from build123d import *

# Parameters (mm, degrees)
SKETCH1_W           = 17
SKETCH1_H           = 18.5
SKETCH1_R           = 1.5
BOSS_EXTRUDE1_DEPTH = 2
SKETCH3_R           = 0.325
LPATTERN1_COUNT     = 4
LPATTERN1_PITCH     = 2.54


with BuildPart() as part:
    # Sketch1 → Boss-Extrude1 (new body)
    with BuildSketch(Plane(origin=(0, 0, 0), x_dir=(1, 0, 0), z_dir=(0, 1, 0))):
        with Locations((8.5, 9.25)):
            Rectangle(SKETCH1_W, SKETCH1_H)
        with Locations(Location((2.5, 15.25, 0), (0, 0, 270))):
            Circle(SKETCH1_R, mode=Mode.SUBTRACT)
        with Locations(Location((2.5, 3.25, 0), (0, 0, 270))):
            Circle(SKETCH1_R, mode=Mode.SUBTRACT)
    extrude(amount=BOSS_EXTRUDE1_DEPTH)

    # Sweep1: sweep along a path in Sketch2
    with BuildLine(Plane.ZY.offset(-7)) as sweep1_path:
        Line((-1, -1), (-1, 3.5))
        ThreePointArc((-1, 3.5), (-0.853553391, 3.853553391), (-0.5, 4))
        Line((-0.5, 4), (29, 4))
    # Sketch3 → Sweep1 (sweep)
    with BuildSketch(Plane(origin=(0, 2, 0), x_dir=(1, 0, 0), z_dir=(0, 1, 0))):
        with Locations((7, 1)):
            Circle(SKETCH3_R)
    sweep1 = sweep(path=sweep1_path.line)

    # LPattern1: Sweep1 ×4
    with Locations(*[(i * LPATTERN1_PITCH, 0, 0) for i in range(1, LPATTERN1_COUNT)]):
        add(sweep1)


solid = part.part
Design review of the part built by this model. Coordinates are the model's own, in mm. Coordinates: 2 decimals unless noted, no trailing zeros. Order: outer loops, then holes, each group sorted by start corner. A loop starts at its lowest first (then second) coordinate and runs counter-clockwise, first axis right, second up. Notation, with made-up numbers: M 9.5,11 L 61.5,11 A27 ccw 61.5,49 Z; hole C -14,-35 d10. An arc over 180 degrees is marked long. Use a Markdown table: item, result.
(1) For P1, Ø3.5, axis at x = 2.5, z = -15.25, coming from the +Y side; P2, Ø1.5, axis at x = 13, z = 23, coming from the +Y side; P3, Ø6, axis at x = 5, z = -4, coming from the -Y side, all flat-tipped, find the tip position at first contact; note any pin that passes through.
Worked answers:
| item | result |
|---|---|
| P1 | stops at y = 2 |
| P2 | stops at y = 4.28 |
| P3 | stops at y = 0 |
(2) Wall thickness on probe 1 along X at (y, z) = (0.55, -3.25); probe 2 along X at (y, z) = (3.95, 7.5); probe 3 along Y at (x, z) = (15, -11): over which ranges is each line inside the solid? List them lowest first.
Worked answers:
| item | result |
|---|---|
| probe 1 | x = 0 to 1, 4 to 17 |
| probe 2 | x = 6.68 to 7.32, 9.22 to 9.86, 11.76 to 12.4, 14.3 to 14.94 |
| probe 3 | y = 0 to 2 |
(3) Add section A-A (x = 3.5). Give the boundary of the cut face in (y, z), then the cut area to 3 significant figures.
Worked answers:
| item | result |
|---|---|
| outline | M 0,-18.5 L 2,-18.5 L 2,-16.37 L 0,-16.37 Z; M 0,-14.13 L 2,-14.13 L 2,-4.37 L 0,-4.37 Z; M 0,-2.13 L 2,-2.13 L 2,0 L 0,0 Z |
| area | 28.1 mm2 |
(4) Add section B-B (z = -15.25). Give the boundary of the cut face in (x, y), then the cut area to 3 significant figures.
Worked answers:
| item | result |
|---|---|
| outline | M 0,0 L 1,0 L 1,2 L 0,2 Z; M 4,0 L 17,0 L 17,2 L 4,2 Z |
| area | 28.0 mm2 |
(5) Add section D-D (x = 7.75). Give the boundary of the cut face in (y, z), then the cut area to 3 significant figures.
Worked answers:
| item | result |
|---|---|
| outline | M 0,-18.5 L 2,-18.5 L 2,0 L 0,0 Z |
| area | 37.0 mm2 |
(6) Add section C-C (z = 25.5). Give the boundary of the cut face in (x, y) (3 decimals), then the cut area to 3 significant figures.
Worked answers:
| item | result |
|---|---|
| outline | C 7,4 d0.65; C 9.54,4 d0.65; C 12.08,4 d0.65; C 14.62,4 d0.65 |
| area | 1.33 mm2 |
(7) Draft analysis for pull direction X (two halves, no side actions). For faces 1 (the flat face through (8, 1, -18.5)), 2 (the flat face through (0, 1, -9)), 3 (the cylindrical face through (1.925, 0.986, -1.864)), 4 (the flat face through (17, 1, -9)), state which applies: released by +X, released by -X, zero draft, split by the parting line, or undercut.
Worked answers:
| item | result |
|---|---|
| face 1 | zero draft |
| face 2 | released by -X |
| face 3 | undercut |
| face 4 | released by +X |
